```python
from build123d import *

# Parameters (mm, degrees)
F1_DEPTH = 12
F2_W     = 55
F2_H     = 20
F3_DEPTH = 20
F5_DEPTH = 25


with BuildPart() as f1:
    # F0 (on Top) → F1 (new body)
    with BuildSketch(Plane.XY):
        Polygon((37.5, 25), (-37.5, 25), (-37.5, -25), (-12.5, -25), (-12.5, -13), (12.5, -13), (12.5, -25), (37.5, -25), align=None)
    extrude(amount=F1_DEPTH)

    # F2 (on face) → F3 (join)
    with BuildSketch(Plane.XY.offset(12)):
        with Locations((10, 15)):
            Rectangle(F2_W, F2_H)
    extrude(amount=F3_DEPTH)

    # F4 (on face) → F5 (cut)
    with BuildSketch(Plane.XZ.offset(-5)):
        Polygon((-17.5, 12), (17.5, 32), (-17.5, 32), align=None)
    extrude(amount=-F5_DEPTH, mode=Mode.SUBTRACT)


solid = f1.part
```
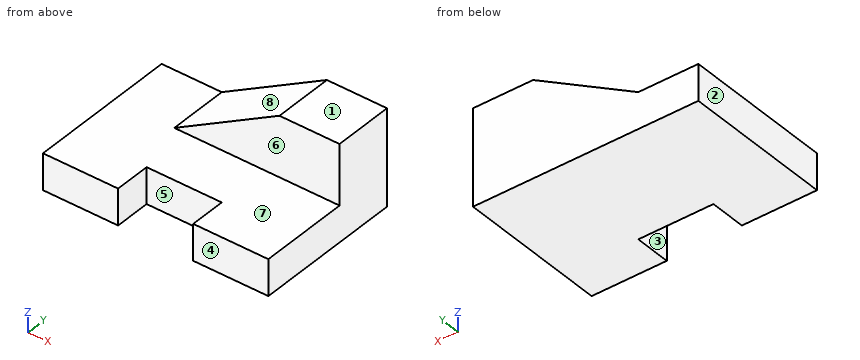
Here's how the part is built. I have some questions about the finished solid (model axes, mm). Face numbers are marked on the shaded views. A direction names the side the tool comes from. Give positions to 0.01 mm unless a question says otherwise; leave off trailing zeros. Write each loop counter-clockwise with the first axis right and the second up, starting at its lowest first coordinate (ties: lowest second). Pieces come first, ordered by that corner, then holes. Notation, with made-up numbers: (47.5, 76) -> (74.5, 76) arc R35 cw to (74.5, 114) -> close; hole circle Ø9 at (50, 77.5). An arc over 180 degrees is marked (long way). Write each question's results on one line, items separated by ' | '.
Item 1: We'd pull the mould along X, two halves only. Please class the marked faces 1, 2 and 3: pulls with the +X half, pulls with the -X half, needs draft (parallel to the pull), parting line crosses it, or undercut.
Output:
face 1: needs draft | face 2: pulls with the -X half | face 3: undercut
Item 2: Suppose I cut it at A-A on z = 10.5. Write out the boundary of the cut face in (x, y).
Output:
outline: (-37.5, -25) -> (-12.5, -25) -> (-12.5, -13) -> (12.5, -13) -> (12.5, -25) -> (37.5, -25) -> (37.5, 25) -> (-37.5, 25) -> close
Item 3: Suppose I cut it at B-B on y = 21. Write out the boundary of the cut face in (x, z).
Output:
outline: (-37.5, 0) -> (37.5, 0) -> (37.5, 32) -> (17.5, 32) -> (-17.5, 12) -> (-37.5, 12) -> close
Item 4: For pin 1 Ø16 at (x, z) = (6.5, 25) entering from -Y; pin 2 Ø13 at (x, z) = (-3, 6) entering from -Y, each with a flat end and sliding along its axis, tell me the tip position at first contact or that it passes through.
Output:
pin 1: stops at y = 5 | pin 2: stops at y = -13
Item 5: On a 3-axis mill with a long thin cutter (end or side, diameter ignored), from which of +Z, -Z, +X, -X, +Y, -Y can I reach the whole of each face in a straight line? I mean the marked faces 4, 5, 6, 7 and 8. Say none if no direction works.
Output:
face 4: +Z, -Z, +X, -X, -Y | face 5: +Z, -Z, -Y | face 6: +Z, +X, -X, -Y | face 7: +Z, -X, -Y | face 8: +Z, -X, +Y, -Y
Item 6: If I drill on L1, parallel to Z at x = 29, y = -3.5; L2, parallel to Y at x = 29, z = 28.5; L3, parallel to Y at x = 10, z = 2, over which ranges is the centre line in solid material (lowest first)?
Output:
L1: z = 0 to 12 | L2: y = 5 to 25 | L3: y = -13 to 25
Item 7: Suppose I cut it at D-D on z = 15. Write out the boundary of the cut face in (x, y).
Output:
outline: (-12.25, 5) -> (37.5, 5) -> (37.5, 25) -> (-12.25, 25) -> close
Item 8: Suppose I cut it at C-C on x = 31. Write out the boundary of the cut face in (y, z), plus the area to 3 significant figures.
Output:
outline: (-25, 0) -> (25, 0) -> (25, 32) -> (5, 32) -> (5, 12) -> (-25, 12) -> close | area: 1,000 mm^2
